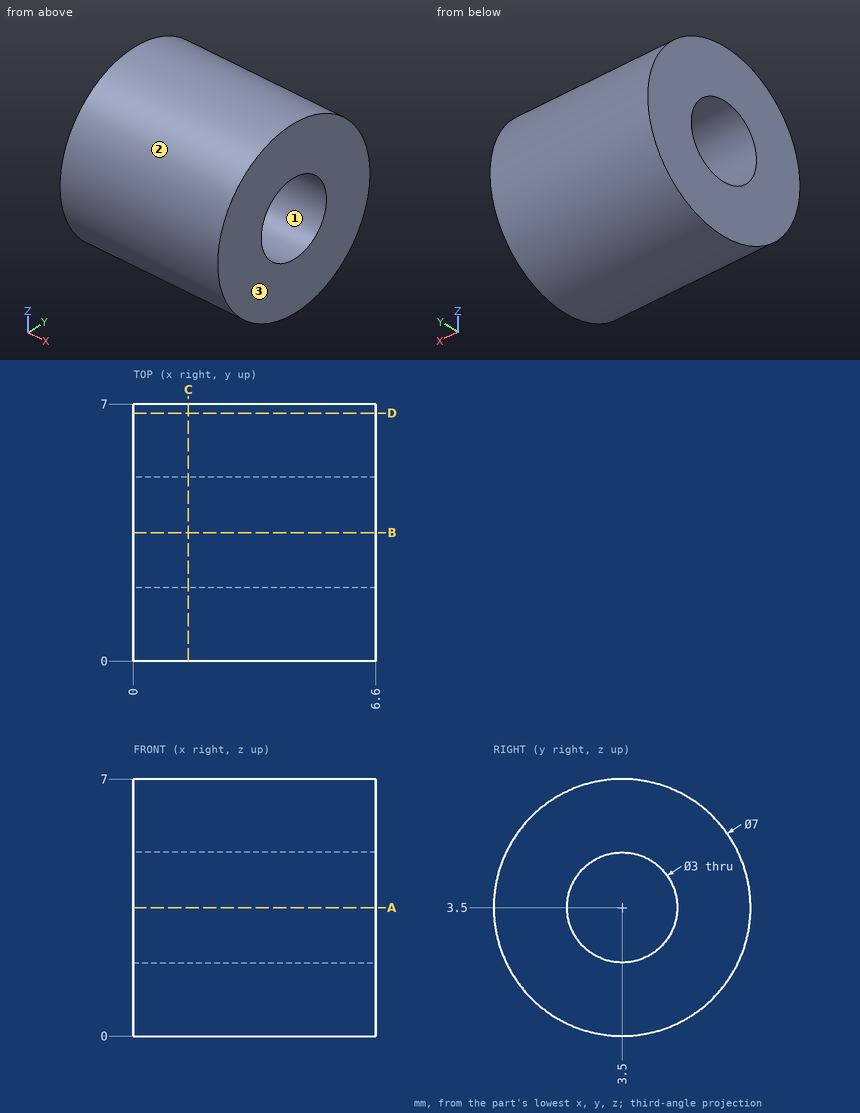
Design review of the part shown in the three views and the two pictorial views. Dimensions are in mm from the part's minimum x, y and z. Coordinates: 2 decimals unless noted, no trailing zeros. Loops run counter-clockwise (first coordinate to the right, second up) from the corner with the lowest first, then second, coordinate; pieces in that order, holes last. Notation, with made-up numbers: M -13.75,-22.75 L 32.25,-22.75 A13 cw 32.25,-1.75 Z; hole C 89.25,10 d11. An arc over 180 degrees is marked long. Put each result on its own line as item: value. Start each with the question number.
Q1. Clearance check with flat-ended pins moving along their axes: pin 1 (1.5 mm diameter, centred on x = 3, z = 1.5, fed in from +Y); pin 2 (1 mm diameter, centred on y = 4.5, z = 5, fed in from -X). State where each tip first meets the part, or that it passes through.
Q2. Add section C-C (x = 1.5). Write out the cut boundary in (y, z).
Q3. Wall thickness on line 1 (Y direction, x = 4.5, z = 3.5); line 2 (Y direction, x = 6.25, z = 4); line 3 (Y direction, x = 2.5, z = 6): over which ranges is each line inside the solid? List them lowest first.
Q4. Add section D-D (y = 6.75). Write out the cut boundary in (x, z), and give its area (3 significant figures).
Q5. Add section A-A (z = 3.5). Write out the cut boundary in (x, y).
Q6. The part is to be moulded in two halves that separate along Z. For the marked faces 1, 2 and 3, say which applies: +Z half, -Z half, draft (parallel to the pull), parting line (faces both ways), or undercut.
Answers:
1. pin 1: stops at y = 6.77
1. pin 2: stops at x = 0
2. outline: C 3.5,3.5 d7; hole C 3.5,3.5 d3
3. line 1: y = 0 to 2, 5 to 7
3. line 2: y = 0.04 to 2.09, 4.91 to 6.96
3. line 3: y = 1.05 to 5.95
4. outline: M 0,2.2 L 6.6,2.2 L 6.6,4.8 L 0,4.8 Z
4. area: 17.1 mm^2
5. outline: M 0,0 L 6.6,0 L 6.6,2 L 0,2 Z; M 0,5 L 6.6,5 L 6.6,7 L 0,7 Z
6. face 1: undercut
6. face 2: parting line
6. face 3: draft
